Here's how the part is built. I have some questions about the finished solid (model axes, mm). Face numbers are marked on the shaded views. Coordinates: 2 decimals unless noted, no trailing zeros. Write each loop counter-clockwise with the first axis right and the second up, starting at its lowest first coordinate (ties: lowest second). Pieces come first, ordered by that corner, then holes. Notation, with made-up numbers: (32.25, 60) -> (85.25, 60) arc R11 ccw to (85.25, 65) -> close; hole circle Ø1 at (50, -24). An arc over 180 degrees is marked (long way). Use a Markdown table: item, result. Add a question column.
Item 1: If we mould it in two halves opening along Y, with no side actions, what happens to the marked faces 1, 2 and 3? For each: pulls with the +Y half, pulls with the -Y half, needs draft (parallel to the pull), parting line crosses it, or undercut.
Item 2: Imagine slicing it at A-A, the plane x = 20.32. Write out the boundary of the cut face in (y, z), and give its area (3 significant figures).
Item 3: Will this pin go through, and if not, where does the flat tip stop? pin 1 Ø8.5 at (x, y) = (11.91, -5.44) entering from -Z.
Item 4: Imagine slicing it at B-B, the plane y = 26.67. Write out the boundary of the cut face in (x, z), and give its area (3 significant figures).
Item 5: Imagine slicing it at C-C, the plane z = 1.5. Count the separate pieces of the cut face and the enclosed holes in it, and give its area (3 significant figures).
Item 6: Imagine slicing it at D-D, the plane x = -12.7. Write out the boundary of the cut face in (y, z), and give its area (3 significant figures).
Item 7: If I drill on line 1 along Y through (x, z) = (27.94, 4.5); line 2 along X through (y, z) = (27, 4.75); line 3 along Y through (x, z) = (30.48, 1.5), over which ranges is the centre line in solid material (lowest first)? Write a range as from..to.
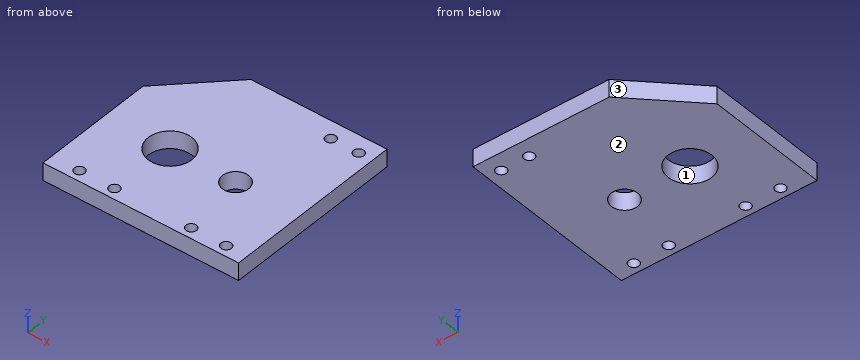
```python
from build123d import *

# Parameters (mm, degrees)
SKETCH1_W             = 71.12
SKETCH1_H             = 66.04
SKETCH1_R             = 7.9375
SKETCH1_R_2           = 4.7625
BOSS_EXTRUDE1_DEPTH   = 6.35
F_6_CLEARANCE_HOLE1_D = 3.7973
CUT_EXTRUDE1_DEPTH    = 49.940336125
F_6_CLEARANCE_HOLE2_D = 3.7973


with BuildPart() as part:
    # Sketch1 → Boss-Extrude1 (new body)
    with BuildSketch(Plane.XY):
        Rectangle(SKETCH1_W, SKETCH1_H)
        with Locations((-11.90625, -5.43814)):
            Circle(SKETCH1_R, mode=Mode.SUBTRACT)
        with Locations((11.90625, -5.43814)):
            Circle(SKETCH1_R_2, mode=Mode.SUBTRACT)
    extrude(amount=BOSS_EXTRUDE1_DEPTH)

    # #6 Clearance Hole1 (through all)
    with Locations(Plane.XY.offset(6.35)):
        with Locations((-25.4, -29.21), (-12.7, -29.21), (15.24, -29.21), (27.94, -29.21)):
            Hole(F_6_CLEARANCE_HOLE1_D / 2)

    # Sketch4 → Cut-Extrude1 (cut, through all)
    with BuildSketch(Plane.XY.offset(6.35)):
        Polygon((-35.56, 11.43), (-35.56, 33.02), (-13.97, 33.02), align=None)
    extrude(amount=-CUT_EXTRUDE1_DEPTH, mode=Mode.SUBTRACT)

    # #6 Clearance Hole2 (through all)
    with Locations(Plane.XY.offset(6.35)):
        with Locations((20.32, 26.67), (30.48, 26.67)):
            Hole(F_6_CLEARANCE_HOLE2_D / 2)


solid = part.part
```
Ans:
| question | item | result |
|---|---|---|
| 1 | face 1 | undercut |
| 1 | face 2 | needs draft |
| 1 | face 3 | pulls with the +Y half |
| 2 | outline | (-33.02, 0) -> (24.77, 0) -> (24.77, 6.35) -> (-33.02, 6.35) -> close; (28.57, 0) -> (33.02, 0) -> (33.02, 6.35) -> (28.57, 6.35) -> close |
| 2 | area | 395 mm^2 |
| 3 | pin 1 | passes through |
| 4 | outline | (-20.32, 0) -> (18.42, 0) -> (18.42, 6.35) -> (-20.32, 6.35) -> close; (22.22, 0) -> (28.58, 0) -> (28.58, 6.35) -> (22.22, 6.35) -> close; (32.38, 0) -> (35.56, 0) -> (35.56, 6.35) -> (32.38, 6.35) -> close |
| 4 | area | 307 mm^2 |
| 5 | separate pieces | 1 |
| 5 | enclosed holes | 8 |
| 5 | area | 4,130 mm^2 |
| 6 | outline | (-33.02, 0) -> (-31.11, 0) -> (-31.11, 6.35) -> (-33.02, 6.35) -> close; (-27.31, 0) -> (-13.34, 0) -> (-13.34, 6.35) -> (-27.31, 6.35) -> close; (2.46, 0) -> (33.02, 0) -> (33.02, 6.35) -> (2.46, 6.35) -> close |
| 6 | area | 295 mm^2 |
| 7 | line 1 | y = -33.02..-31.11, -27.31..33.02 |
| 7 | line 2 | x = -19.99..18.45, 22.19..28.61, 32.35..35.56 |
| 7 | line 3 | y = -33.02..24.77, 28.57..33.02 |
